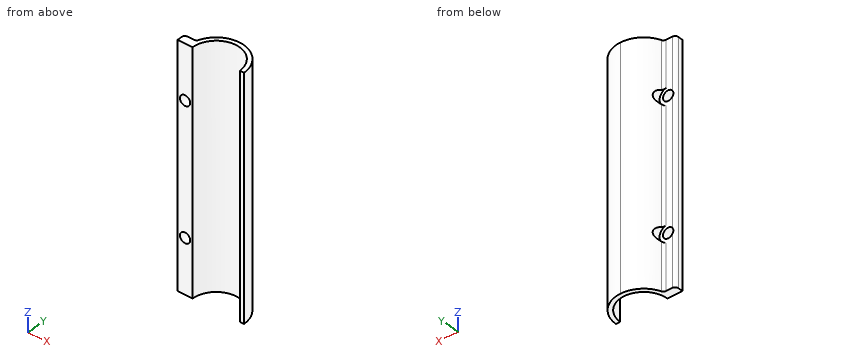
```python
from build123d import *

# Parameters (mm, degrees)
BOSS_EXTRUDE1_DEPTH           = 112
SKETCH6_W                     = 2.4
SKETCH6_H                     = 3.81
M4_CLEARANCE_HOLE2_AT_2_COUNT = 2
M4_CLEARANCE_HOLE2_AT_2_PITCH = 61.2
SKETCH7_R                     = 4
CUT_EXTRUDE1_DEPTH            = 114.80885774
FILLET1_R                     = 1.5


with BuildPart() as part:
    # Sketch1 → Boss-Extrude1 (new body)
    with BuildSketch(Plane.XY):
        with BuildLine():
            ThreePointArc((-12.429155241, 3.81), (-12.856496765, 1.926263465), (-13, 0))
            Line((-13, 0), (-11, 0))
            ThreePointArc((-11, 0), (0, 11), (11, 0))
            Line((11, 0), (13, 0))
            ThreePointArc((13, 0), (9.192388155, 9.192388155), (0, 13))
            ThreePointArc((0, 13), (-7.728842087, 10.452990003), (-12.429155241, 3.81))
        make_face()
        with BuildLine():
            Line((-18, 0), (-13, 0))
            ThreePointArc((-13, 0), (-12.856496765, 1.926263465), (-12.429155241, 3.81))
            Line((-12.429155241, 3.81), (-18, 3.81))
            Line((-18, 3.81), (-18, 0))
        make_face()
    extrude(amount=BOSS_EXTRUDE1_DEPTH)

    # Sketch6 → M4 Clearance Hole2 (revolve, cut)
    with BuildSketch(Plane(origin=(-14.5, 3.81, 86.6), x_dir=(0, 0, 1), z_dir=(1, 0, 0))):
        with Locations((1.2, 1.905)):
            Rectangle(SKETCH6_W, SKETCH6_H)
    m4_clearance_hole2 = revolve(axis=Axis((-14.5, 10.16, 86.6), (0, -1, 0)), mode=Mode.SUBTRACT)

    # M4 Clearance Hole2 at 2: M4 Clearance Hole2 ×2
    with Locations(*[(0, 0, -i * M4_CLEARANCE_HOLE2_AT_2_PITCH) for i in range(1, M4_CLEARANCE_HOLE2_AT_2_COUNT)]):
        add(m4_clearance_hole2, mode=Mode.SUBTRACT)

    # Sketch7 → Cut-Extrude1 (cut, through all)
    with BuildSketch(Plane(origin=(0, 3.81, 0), x_dir=(1, 0, 0), z_dir=(0, 1, 0))):
        with Locations((-14.5, -25.4)):
            Circle(SKETCH7_R)
        with Locations((-14.5, -86.6)):
            Circle(SKETCH7_R)
    extrude(amount=CUT_EXTRUDE1_DEPTH, mode=Mode.SUBTRACT)

    # Fillet1
    # the kernel refuses this fillet: 1.5 mm, written as the material it adds along each edge
    with BuildSketch(Plane(origin=(-12.429155241, 3.81, 87.363272187), x_dir=(0.32988946400333646, 0.9440195662906523, 0), z_dir=(0, 0, 1))) as fillet1_piece_1_section:
        with BuildLine():
            CenterArc((1.065165566, 1.498874377), FILLET1_R, 199.262066546, 68.518123934)
            Line((-0.350863784, 1.004040181), (0, 0))
            ThreePointArc((0, 0), (0.503532813, 0.009755402), (1.007065626, 0))
        make_face()
    fillet1_piece_1 = extrude(amount=24.636727813, mode=Mode.PRIVATE)
    fillet1_piece_1 = fillet1_piece_1 - Plane(origin=(-14.5, 4.019727469, 86.6), x_dir=(1, 0, 0), z_dir=(0, -1, 0)) * Cylinder(4, 54, mode=Mode.PRIVATE)
    add(fillet1_piece_1)
    with BuildSketch(Plane(origin=(-12.429155241, 3.81, 26.163272187), x_dir=(0.32988946400333646, 0.9440195662906523, 0), z_dir=(0, 0, 1))) as fillet1_piece_2_section:
        with BuildLine():
            CenterArc((1.065165566, 1.498874377), FILLET1_R, 199.262066546, 68.518123934)
            Line((-0.350863784, 1.004040181), (0, 0))
            ThreePointArc((0, 0), (0.503532813, 0.009755402), (1.007065626, 0))
        make_face()
    fillet1_piece_2 = extrude(amount=59.673455626, mode=Mode.PRIVATE)
    fillet1_piece_2 = fillet1_piece_2 - Plane(origin=(-14.5, 4.019506005, 86.6), x_dir=(1, 0, 0), z_dir=(0, -1, 0)) * Cylinder(4, 124, mode=Mode.PRIVATE)
    fillet1_piece_2 = fillet1_piece_2 - Plane(origin=(-14.5, 4.019506005, 25.4), x_dir=(1, 0, 0), z_dir=(0, -1, 0)) * Cylinder(4, 124, mode=Mode.PRIVATE)
    add(fillet1_piece_2)
    with BuildSketch(Plane(origin=(-12.429155241, 3.81, 0), x_dir=(0.3298894640033357, 0.9440195662906526, 0), z_dir=(0, 0, 1))) as fillet1_piece_3_section:
        with BuildLine():
            CenterArc((1.065165566, 1.498874377), FILLET1_R, 199.262066546, 68.518123934)
            Line((-0.350863784, 1.004040181), (0, 0))
            ThreePointArc((0, 0), (0.503532813, 0.009755402), (1.007065626, 0))
        make_face()
    fillet1_piece_3 = extrude(amount=24.636727813, mode=Mode.PRIVATE)
    fillet1_piece_3 = fillet1_piece_3 - Plane(origin=(-14.5, 4.019727315, 25.4), x_dir=(1, 0, 0), z_dir=(0, -1, 0)) * Cylinder(4, 54, mode=Mode.PRIVATE)
    add(fillet1_piece_3)
    # the kernel refuses this fillet: 1.5 mm, written as the material it takes off along each edge
    with BuildSketch(Plane(origin=(-18, 3.81, -3.75), x_dir=(1, 0, 0), z_dir=(0, 0, 1))) as fillet1_2_piece_1:
        with BuildLine():
            CenterArc((FILLET1_R, -FILLET1_R), FILLET1_R, 90, 90)
            Line((0, -FILLET1_R), (0, 0))
            Line((0, 0), (FILLET1_R, 0))
        make_face()
    extrude(amount=119.5, mode=Mode.SUBTRACT)


solid = part.part
```
Geometry check sheet. Reference: the model listing, model coordinates, mm. Coordinates: 2 decimals unless noted, no trailing zeros. Order: outer loops, then holes, each group sorted by start corner. A loop starts at its lowest first (then second) coordinate and runs counter-clockwise, first axis right, second up. Notation, with made-up numbers: (-13, -2.5) - (45, -2.5) arc R18 cw to (45, 12.5) - close; hole circle Ø3 at (20, -27.75). An arc over 180 degrees is marked (long way). Answer as a JSON object with one key per item and string values. Group by question number.
Item 1: Sectioned sample at C-C, the plane y = 6. Record the cut outline in (x, z).
Item 2: Sectioned sample at B-B, the plane z = 86.6. Record the cut outline in (x, y), and give its area (3 significant figures).
Item 3: Depth check by flat-ended pin: pin 1 Ø2 at (y, z) = (7, 92) entering from +X; pin 2 Ø6.5 at (x, z) = (-15, 57.5) entering from +Y; pin 3 Ø6 at (x, z) = (1.5, 50) entering from -Y; pin 4 Ø6 at (x, z) = (-14.5, 25.4) entering from -Y. Enter the tip coordinate at first touch or a pass-through.
Item 4: Scan lines: probe 1 along X at (y, z) = (1.9, 86.6); probe 2 along X at (y, z) = (2.8, 86.6); probe 3 along Y at (x, z) = (-14, 34.5). Record each from-to range of solid material in increasing order.
Item 5: Sectioned sample at A-A, the plane x = -14.5. Record the cut outline in (y, z).
Item 6: Sectioned sample at D-D, the plane x = 1. Record the cut outline in (y, z), and give its area (3 significant figures).
Resolved:
{
 "1": {"outline": "(-11.53, 0) - (-9.22, 0) - (-9.22, 112) - (-11.53, 112) - (-11.53, 89.28) arc R4 cw to (-11.53, 83.92) - (-11.53, 28.08) arc R4 cw to (-11.53, 22.72) - close; (9.22, 0) - (11.53, 0) - (11.53, 112) - (9.22, 112) - close"},
 "2": {"outline": "(-18, 0) - (-16.9, 0) - (-16.9, 3.76) arc R1.5 ccw to (-18, 2.31) - close; (-12.1, 0) - (-11, 0) arc R11 cw to (11, 0) - (13, 0) arc R13 ccw to (-10.5, 7.66) - (-10.5, 3.81) - (-12.1, 3.81) - close", "area": "72.2 mm^2"},
 "3": {"pin 1": "x = 11.53", "pin 2": "y = 5.56", "pin 3": "y = 10.04", "pin 4": "y = 0"},
 "4": {"probe 1": "-18 to -16.9, -12.1 to -10.83, 10.83 to 12.86", "probe 2": "-17.92 to -16.9, -12.1 to -10.64, 10.64 to 12.69", "probe 3": "0 to 3.81"},
 "5": {"outline": "(0, 0) - (3.81, 0) - (3.81, 23) - (0, 23) - close; (0, 27.8) - (3.81, 27.8) - (3.81, 84.2) - (0, 84.2) - close; (0, 89) - (3.81, 89) - (3.81, 112) - (0, 112) - close"},
 "6": {"outline": "(10.95, 0) - (12.96, 0) - (12.96, 112) - (10.95, 112) - close", "area": "225 mm^2"}
}
